Can you work these out from the model? Positions are in its coordinate system, mm. A direction names the side the tool comes from. Coordinates: 2 decimals unless noted, no trailing zeros. Write each loop counter-clockwise with the first axis right and the second up, starting at its lowest first coordinate (ties: lowest second). Pieces come first, ordered by that corner, then holes. Notation, with made-up numbers: (20, -26.75) -> (31, -26.75) arc R14 ccw to (31, -3.75) -> close; hole circle Ø3 at (-33, 35.25). An arc over 180 degrees is marked (long way). Use one line per item in the form item = value.
```python
from build123d import *

# Parameters (mm, degrees)
SKETCH_1_R          = 7.5
SKETCH_1_R_2        = 4.35
EXTRUDE_1_DEPTH     = 17
SKETCH_3_R          = 6
CUT_EXTRUDE_2_DEPTH = 3
SKETCH_4_R          = 7.5
EXTRUDE_3_DEPTH     = 8
SKETCH_5_R          = 1.25
CUT_EXTRUDE_4_DEPTH = 13.5
SKETCH_6_R          = 4.5
CUT_EXTRUDE_5_DEPTH = 4.5
SKETCH_7_R          = 4.5
CUT_EXTRUDE_6_DEPTH = 2.5
CUT_EXTRUDE_6_DRAFT = -50
EXTRUDE_START       = -8
SKETCH_8_R          = 15
SKETCH_8_R_2        = 7.5
EXTRUDE_8_DEPTH     = 8
FILLET_1_R          = 3


with BuildPart() as part:
    # Эскиз1 → Вытянуть1 (new body)
    with BuildSketch(Plane.XY):
        Circle(SKETCH_1_R)
        Circle(SKETCH_1_R_2, mode=Mode.SUBTRACT)
    extrude(amount=EXTRUDE_1_DEPTH)

    # Эскиз3 → Вытянуть2 (cut)
    with BuildSketch(Plane(origin=(0, 0, 0), x_dir=(-1, 0, 0), z_dir=(0, 0, -1))):
        Circle(SKETCH_3_R)
    extrude(amount=-CUT_EXTRUDE_2_DEPTH, mode=Mode.SUBTRACT)

    # Эскиз4 → Вытянуть3 (add)
    with BuildSketch(Plane.XY.offset(17)):
        Circle(SKETCH_4_R)
    extrude(amount=EXTRUDE_3_DEPTH)

    # Эскиз5 → Вытянуть4 (cut, symmetric)
    with BuildSketch(Plane.XY.offset(25)):
        Circle(SKETCH_5_R)
    extrude(amount=CUT_EXTRUDE_4_DEPTH, both=True, mode=Mode.SUBTRACT)

    # Эскиз6 → Вытянуть5 (cut)
    with BuildSketch(Plane.XY.offset(25)):
        Circle(SKETCH_6_R)
    extrude(amount=-CUT_EXTRUDE_5_DEPTH, mode=Mode.SUBTRACT)


with BuildPart() as cut_extrude_6_tool:
    # Эскиз7 → Вытянуть6 (with draft: the straight prism first)
    with BuildSketch(Plane.XY.offset(20.5)):
        Circle(SKETCH_7_R)
    extrude(amount=-CUT_EXTRUDE_6_DEPTH)
    # Вытянуть6: the draft: its side faces are tilted about the plane it starts from
    cut_extrude_6_sides = [cut_extrude_6_tool.faces().sort_by_distance(p)[0] for p in [
        (-4.5, 0, 19.25),
    ]]
    draft(cut_extrude_6_sides, Plane.XY.offset(20.5), CUT_EXTRUDE_6_DRAFT)


with BuildPart() as part_1:
    add(part.part)

    # Вытянуть6: cut by cut_extrude_6_tool
    add(cut_extrude_6_tool.part, mode=Mode.SUBTRACT)

    # Эскиз8 → Вытянуть8 (add)
    with BuildSketch(Plane.XY.offset(25).offset(EXTRUDE_START)):
        Circle(SKETCH_8_R)
        Circle(SKETCH_8_R_2, mode=Mode.SUBTRACT)
    extrude(amount=EXTRUDE_8_DEPTH)

    # Скругление1
    fillet_1_edges = [part_1.edges().sort_by_distance(p)[0] for p in [
        (-7.5, 0, 17),
    ]]
    fillet(fillet_1_edges, radius=FILLET_1_R)


solid = part_1.part
```
Q1. Thinking about a two-plate mould opening in X: for faces 3 (the cylindrical face through (-0.59, 4.46, 22.78)), 4 (the flat face through (3, 4, 25)), 5 (the cylindrical face through (-14.985, 0.66, 20.944)), which applies, released by +X, released by -X, zero draft, split by the parting line, or undercut?
Return value:
face_3 = undercut
face_4 = zero draft
face_5 = split by the parting line
Q2. Suppose I cut it at A-A (x = 0). Write out the boundary of the cut face in (y, z), then the cut area to 3 significant figures.
Return value:
outline = (-15, 17) -> (-10.5, 17) arc R3 cw to (-7.5, 14) -> (-7.5, 0) -> (-6, 0) -> (-6, 3) -> (-4.35, 3) -> (-4.35, 17) -> (-1.25, 17) -> (-1.25, 18) -> (-1.52, 18) -> (-4.5, 20.5) -> (-4.5, 25) -> (-15, 25) -> close; (1.25, 17) -> (4.35, 17) -> (4.35, 3) -> (6, 3) -> (6, 0) -> (7.5, 0) -> (7.5, 14) arc R3 cw to (10.5, 17) -> (15, 17) -> (15, 25) -> (4.5, 25) -> (4.5, 20.5) -> (1.52, 18) -> (1.25, 18) -> close
area = 283 mm2
Q3. Will these pins go through, and if not, where does the flat tip stop? pin 1 (12 mm diameter, centred on x = -11.5, z = 3.5, fed in from -Y); pin 2 (5 mm diameter, centred on y = 4, z = 8.5, fed in from +X); pin 3 (12 mm diameter, centred on y = 9.5, z = 9, fed in from +X); pin 4 (2 mm diameter, centred on x = 0, y = 0, fed in from -Z) (3 decimals).
Return value:
pin_1 = -5.1
pin_2 = 7.35
pin_3 = 6.63
pin_4 = through
Q4. Suppose I cut it at C-C (z = 2.25). Write out the boundary of the cut face in (x, y).
Return value:
outline = circle Ø15 at (0, 0); hole circle Ø12 at (0, 0)
Q5. If I drill on line 1 (Y direction, x = 0, z = 1.35); line 2 (Y direction, x = 0, z = 9); line 3 (X direction, y = -1.25, z = 5.25), over which ranges is the centre line in solid material (lowest first)? Write a range as from..to.
Return value:
line_1 = -7.5..-6, 6..7.5
line_2 = -7.5..-4.35, 4.35..7.5
line_3 = -7.4..-4.17, 4.17..7.4
Q6. Suppose I cut it at D-D (z = 14.75). Write out the boundary of the cut face in (x, y), then the cut area to 3 significant figures.
Return value:
outline = circle Ø15.19 at (0, 0); hole circle Ø8.7 at (0, 0)
area = 122 mm2
Q7. For faces 1 (the flat face through (3.1, 10.2, 17)), 2 (the conical face through (-0.37, -1.67, 18.16)), which set-ups out of +Z, -Z, +X, -X, +Y, -Y let a thin tool reach every point of the face, with its end or its side?
Return value:
face_1 = -Z
face_2 = +Z
